from build123d import *


with BuildPart() as part:
    # Sweep1: sweep along a path in Sketch1
    with BuildLine(Plane(origin=(0, 0, 0), x_dir=(1, 0, 0), z_dir=(0, 1, 0))) as sweep1_path:
        Line((0, 0), (0, 36))
        Line((0, 36), (-36, 36))
    # Sketch2 → Sweep1 (sweep)
    with BuildSketch(Plane.XY):
        Polygon((0, 0), (0, 23), (3, 23), (3, 3), (42.37, 3), (42.37, 23), (45.37, 23), (45.37, 0), align=None)
    sweep(path=sweep1_path.line, transition=Transition.RIGHT)


solid = part.part
Verification items for the finished model (mm, model axes). A direction names the side the tool comes from. Give positions to 0.01 mm unless a question says otherwise; leave off trailing zeros. Loops run counter-clockwise (first coordinate to the right, second up) from the corner with the lowest first, then second, coordinate; pieces in that order, holes last.
1. Cross-section at C-C on z = -31.5. Record the cut outline in (x, y), and give its area (3 significant figures).
Derived:
outline: (0, 0) - (45.37, 0) - (45.37, 23) - (42.37, 23) - (42.37, 3) - (3, 3) - (3, 23) - (0, 23) - close
area: 256 mm2
2. Cross-section at D-D on z = -50. Record the cut outline in (x, y).
Derived:
outline: (-36, 0) - (45.37, 0) - (45.37, 23) - (42.37, 23) - (42.37, 3) - (-36, 3) - close
3. Release check for a two-part mould opening along X. For faces 4 (the flat face through (24, 2, 0)), 5 (the flat face through (42.37, 13, -40)), 6 (the flat face through (0, 12, -18)), 7 (the flat face through (3, 13, -20)) record: +X half, -X half, draft (parallel to the pull), parting line (faces both ways), or undercut.
Derived:
face 4: draft
face 5: undercut
face 6: -X half
face 7: undercut
4. Cross-section at A-A on y = 16.5. Record the cut outline in (x, z), and give its area (3 significant figures).
Derived:
outline: (-36, -81.37) - (45.37, -81.37) - (45.37, 0) - (42.37, 0) - (42.37, -78.37) - (-36, -78.37) - close; (-36, -39) - (3, -39) - (3, 0) - (0, 0) - (0, -36) - (-36, -36) - close
area: 704 mm2
5. Cross-section at B-B on x = -10. Record the cut outline in (y, z), and give its area (3 significant figures).
Derived:
outline: (0, -81.37) - (23, -81.37) - (23, -78.37) - (3, -78.37) - (3, -39) - (23, -39) - (23, -36) - (0, -36) - close
area: 256 mm2
6. Material ranges on probe 1 along Z at (x, y) = (-5.5, 5); probe 2 along X at (y, z) = (7.25, -11.5); probe 3 along X at (y, z) = (16.25, -36.5), recorded low to high.
Derived:
probe 1: z = -81.37 to -78.37, -39 to -36
probe 2: x = 0 to 3, 42.37 to 45.37
probe 3: x = -36 to 3, 42.37 to 45.37
7. Go/stop test with flat-tipped pins: P1, Ø10, axis at y = 9, z = -11, coming from the -X side; P2, Ø5, axis at x = 31.5, z = -49.5, coming from the +Y side; P3, Ø3, axis at y = 16, z = -52, coming from the -X side. Record where each tip stops, or that it passes through.
Derived:
P1: stops at x = 0
P2: stops at y = 3
P3: stops at x = 42.37
8. Tool access check on faces 1 (the flat face through (-17, 13, -39)), 2 (the flat face through (1, 23, -28)), 3 (the flat face through (-18, 12, -36)). Record the directions out of +Z, -Z, +X, -X, +Y, -Y that give a thin tool (end or side, any length) a straight path to the whole face; none if there is none.
Derived:
face 1: -X, +Y
face 2: +Z, -Z, +X, -X, +Y
face 3: +Z, -X, +Y, -Y
